Design review of the part built by this model. Coordinates are the model's own, in mm. A direction names the side the tool comes from. Round coordinates to 2 decimals unless told otherwise and drop trailing zeros. One line per question, with ' | ' between items. Start each with the question number.
1) Insertion check: pin 1 Ø3.5 at (x, y) = (0.5, 0) entering from -Z; pin 2 Ø2 at (y, z) = (2, -2) entering from -X; pin 3 Ø1 at (x, z) = (2, -7) entering from -Y. Each pin has a flat end and moves straight along its axis. Give the tip position at first contact, or say it passes through.
2) Mouldability with a two-part tool opening along X and no side actions: class faces 4 (the cylindrical face through (3.997, 0.161, -0.606)), 5 (the flat face through (2, 3, 0)), 6 (the flat face through (0, 2, -12.45)) as +X half, -X half, draft (parallel to the pull), parting line (faces both ways), or undercut.
3) For faces 1 (the cylindrical face through (-3, -0.1, 0.2)), 2 (the flat face through (2, 0, -12.45)), 3 (the cylindrical face through (-4.01, 0.01, -0.6)), list the 3-axis set-ups (+Z, -Z, +X, -X, +Y, -Y) from which the entire face can be reached by the end or side of a thin tool; tool diameter is ignored.
4) For probe 1 along Z at (x, y) = (0.75, 3.5); probe 2 along Z at (x, y) = (-1.5, -1.5); probe 3 along Z at (x, y) = (-3, -2.5), list the stretches that pass through material, from the lowest coordinate up.
Autodesk Inventor part; units mm, degrees
ref_plane "YZ Plane" through (0, 0, 0) normal (1, 0, 0) x (0, 1, 0)
ref_plane "XZ Plane" through (0, 0, 0) normal (0, 1, 0) x (-1, 0, 0)
ref_plane "XY Plane" through (0, 0, 0) normal (0, 0, 1) x (1, 0, 0)
sketch "Sketch1" plane through (0, 0, 0) normal (0, 1, 0) x (-1, 0, 0)
  line L0 (0, 0) -> (3.8, 0)
  line L1 (4, -0.2) -> (4, -1)
  arc A0 (4, -1) -> (4, -2) centre (4.2887, -1.5) ccw
  line L2 (4, -2) -> (4, -12.3)
  line L3 (3.8, -12.5) -> (0, -12.5)
  line L4 (0, -12.5) -> (0, 0)
  line L5 (4, -1) -> (3.134, -1.5) construction
  arc A1 (3.8, -12.5) -> (4, -12.3) centre (3.8, -12.3) ccw
  arc A2 (4, -0.2) -> (3.8, 0) centre (3.8, -0.2) ccw
  line L6 (0, -12.5) -> (0, -12.51)
  line L7 (0, -12.51) -> (3.8, -12.51)
  arc A3 (3.8, -12.51) -> (4.01, -12.3) centre (3.8, -12.3) ccw
  line L8 (4.01, -12.3) -> (4.01, -1.9942)
  arc A4 (4.01, -1.0058) -> (4.01, -1.9942) centre (4.2887, -1.5) ccw
  line L9 (4.01, -1.0058) -> (4.01, -0.2)
  arc A5 (4.01, -0.2) -> (3.864, 0) centre (3.8, -0.2) ccw
  line L10 (3.864, 0) -> (3.8, 0)
  line L11 (3.7113, -1.5) -> (3.7213, -1.5) construction
  point P0 (4, 0)
  point P1 (4, -12.5)
  dimension "d0" = 4
  dimension "d1" = 12.5
  dimension "d3" = 1
  dimension "d4" = 60
  dimension "d5" = 1
  dimension "d7" = 0.2
  dimension "d8" = 0.2
  dimension "d20" = 0.01
revolve "Revolution1" add sketch "Sketch1" angle 360 about axis through (0, 0, -12.5) along (0, 0, 1) contours L0 A2 L1 A0 L2 A1 L3 L4
revolve "Revolution2" add sketch "Sketch1" angle 30 mid plane about axis through (0, 0, -12.5) along (0, 0, 1) contours L10 A5 L9 A4 L8 A3 L7 L6 L3 A1 L2 A0 L1 A2
sketch "Sketch2" plane through (0, 0, -12.5) normal (0, 0, -1) x (-1, 0, 0)
  circle A0 centre (0, 0) radius 3
  dimension "d9" = 6
extrude "Extrusion1" cut sketch "Sketch2" against normal mid plane 0.1
sketch "Sketch6" plane through (0, 0, 0) normal (0, 0, 1) x (1, 0, 0)
  circle A0 centre (0, 0) radius 3
  dimension "d27" = 6
extrude "Extrusion4" add sketch "Sketch6" along normal blind 0.5
sketch "Sketch3" plane through (0, 0, 0.5) normal (0, 0, 1) x (1, 0, 0)
  circle A0 centre (-1.75, 0) radius 0.3
  circle A1 centre (1.75, 0) radius 0.3
  line L0 (0, -5.6) -> (0, 5.6) construction
  point P0 (0, 0)
  dimension "d12" = 3.5
  dimension "d13" = 0.6
extrude "Extrusion2" add sketch "Sketch3" along normal blind 2
sketch "Sketch5" plane through (0, 0, -12.45) normal (0, 0, -1) x (-1, 0, 0)
  line L0 (-2.0126, 2.2247) -> (0, 0.2121)
  line L1 (0, 0.2121) -> (2.0126, 2.2247)
  circle A0 centre (0, 0) radius 3
  line L2 (-2.2247, 2.0126) -> (-0.2121, 0)
  line L3 (-0.2121, 0) -> (-2.2247, -2.0126)
  line L4 (-2.0126, -2.2247) -> (0, -0.2121)
  line L5 (0, -0.2121) -> (2.0126, -2.2247)
  line L6 (2.2247, -2.0126) -> (0.2121, 0)
  line L7 (0.2121, 0) -> (2.2247, 2.0126)
  line L8 (0, 0.2121) -> (0.2121, 0) construction
  line L9 (0, -0.2121) -> (-0.2121, 0) construction
  line L10 (-0.2121, 0) -> (0, 0.2121) construction
  line L11 (0, -0.2121) -> (0.2121, 0) construction
  dimension "d23" = 0.3
extrude "Extrusion3" cut sketch "Sketch5" against normal blind 0.1 contours L0 L1 A0 L7 L6 L5 L4 L3 L2
fillet "Fillet1" radius 0.2 4 edges at (0, 0.2121, -12.4) (-0.2121, 0, -12.4) (0, -0.2121, -12.4) (0.2121, 0, -12.4)
properties part number "CPOL-D8-H11_5-P3_5"
From the geometry:
1) pin 1: stops at z = -12.45 | pin 2: stops at x = -3.88 | pin 3: stops at y = -3.71
2) face 4: parting line | face 5: draft | face 6: undercut
3) face 1: +Z | face 2: -Z | face 3: +Z, -Z, -X
4) probe 1: z = -12.5 to 0 | probe 2: z = -12.35 to 0.5 | probe 3: z = -12.47 to -1.93, -1.07 to -0.03
